from build123d import *

# Parameters (mm, degrees)
F0_R     = 1.75
F1_DEPTH = 13
F2_DEPTH = 6
F3_DEPTH = 20
F4_R     = 2.1
F5_DEPTH = 25


with BuildPart() as f1:
    # F0 (on Front) → F1 (new body)
    with BuildSketch(Plane.XZ):
        with BuildLine():
            ThreePointArc((-12, -7.4), (-6.76741, -5.23259), (-4.6, 0))
            ThreePointArc((-4.6, 0), (-6.76741, 5.23259), (-12, 7.4))
            ThreePointArc((-12, 7.4), (-19.4, 0), (-12, -7.4))
        make_face()
        with Locations((-12, 0)):
            Circle(F0_R, mode=Mode.SUBTRACT)
    extrude(amount=-F1_DEPTH)

    # F0 (on Front) → F2 (join)
    with BuildSketch(Plane.XZ):
        with BuildLine():
            ThreePointArc((-12, 7.4), (-6.76741, 5.23259), (-4.6, 0))
            ThreePointArc((-4.6, 0), (-6.76741, -5.23259), (-12, -7.4))
            Line((-12, -7.4), (0, -7.4))
            Line((0, -7.4), (0, 0))
            Line((0, 0), (0, 7.4))
            Line((0, 7.4), (-12, 7.4))
        make_face()
        Polygon((6, 7.4), (0, 7.4), (0, 0), (0, -7.4), (6, -7.4), align=None)
    extrude(amount=-F2_DEPTH)

    # F0 (on Front) → F3 (join)
    with BuildSketch(Plane.XZ):
        Polygon((6, 7.4), (0, 7.4), (0, 0), (0, -7.4), (6, -7.4), align=None)
    extrude(amount=F3_DEPTH)

    # F4 (on Right) → F5 (cut)
    with BuildSketch(Plane.YZ):
        with Locations((-12, 0)):
            Circle(F4_R)
        with Locations((-4, 0)):
            Circle(F4_R)
    extrude(amount=F5_DEPTH, mode=Mode.SUBTRACT)


solid = f1.part
The model under review builds one solid part; all positions refer to its coordinate system, in mm. A direction names the side the tool comes from. Coordinates: 2 decimals unless noted, no trailing zeros. Loops run counter-clockwise (first coordinate to the right, second up) from the corner with the lowest first, then second, coordinate; pieces in that order, holes last. Notation, with made-up numbers: M 12,30.25 L 24,30.25 A15 cw 24,51.25 Z; hole C 18,-19 d1. An arc over 180 degrees is marked long. Put each result on its own line as item: value. Start each with the question number.
Q1. Clearance check with flat-ended pins moving along their axes: pin 1 (5 mm diameter, centred on x = -7, y = 9, fed in from +Z); pin 2 (4.5 mm diameter, centred on x = 1, z = 2, fed in from +Y); pin 3 (7.5 mm diameter, centred on y = -6, z = -2.5, fed in from -X). State where each tip first meets the part, or that it passes through.
Q2. Wall thickness on line 1 (Z direction, x = -12, y = 3.5); line 2 (Y direction, x = 1.5, z = 0.5); line 3 (Z direction, x = 2.2, y = -4): over which ranges is each line inside the solid? List them lowest first.
Q3. The part is to be moulded in two halves that separate along Y. For faces 1 (the flat face through (1, -4, 7.4)), 2 (the cylindrical face through (2.96, -14.1, 0.09)), 3 (the flat face through (-12, 13, 2)), 4 (the flat face through (3, -20, 0)), say which applies: +Y half, -Y half, draft (parallel to the pull), parting line (faces both ways), or undercut.
Q4. Add section D-D (z = -0.5). Write out the cut boundary in (x, y).
Q5. Add section C-C (x = 2). Write out the cut boundary in (y, z).
Q6. Add section A-A (y = -12). Write out the cut boundary in (x, z), and give its area (3 significant figures).
Q7. For faces 5 (the flat face through (0, -10, 2)), 6 (the cylindrical face through (-10.331, 6.409, 0.526)), list the 3-axis set-ups (+Z, -Z, +X, -X, +Y, -Y) from which the entire face can be reached by the end or side of a thin tool; tool diameter is ignored.
Answers:
1. pin 1: stops at z = 6.96
1. pin 2: stops at y = 6
1. pin 3: stops at x = 0
2. line 1: z = -7.4 to -1.75, 1.75 to 7.4
2. line 2: y = -20 to -14.04, -9.96 to -6.04, -1.96 to 6
2. line 3: z = -7.4 to -2.1, 2.1 to 7.4
3. face 1: draft
3. face 2: undercut
3. face 3: +Y half
3. face 4: -Y half
4. outline: M -19.38,0 L -13.68,0 L -13.68,13 L -19.38,13 Z; M -10.32,0 L 0,0 L 0,-1.96 L 6,-1.96 L 6,6 L -4.62,6 L -4.62,13 L -10.32,13 Z; M 0,-20 L 6,-20 L 6,-14.04 L 0,-14.04 Z; M 0,-9.96 L 6,-9.96 L 6,-6.04 L 0,-6.04 Z
5. outline: M -20,-7.4 L 6,-7.4 L 6,7.4 L -20,7.4 Z; hole C -12,0 d4.2; hole C -4,0 d4.2
6. outline: M 0,-7.4 L 6,-7.4 L 6,-2.1 L 0,-2.1 Z; M 0,2.1 L 6,2.1 L 6,7.4 L 0,7.4 Z
6. area: 63.6 mm^2
7. face 5: +Z, -Z, -X, -Y
7. face 6: +Y, -Y
